The listing builds one solid part. Answer for the finished solid, in the listing's coordinates (mm). Face numbers are marked on the shaded views. A direction names the side the tool comes from. Round coordinates to 2 decimals unless told otherwise and drop trailing zeros.
(1) Find the intervals of material crossed by probe 1 along Y at (x, z) = (5, -12.5); probe 2 along Z at (x, y) = (5, -8.5); probe 3 along Y at (x, z) = (4.5, -1.5), in increasing order.
(2) A cutting plane is placed at A-A, the plane x = 4. Give the number of separate pieces and of enclosed holes in the cut face, and give its area (3 significant figures).
(3) For the marked faces 1 and 2, determine the directions among +Z, -Z, +X, -X, +Y, -Y from which every point of the face is accessible in a straight line to the end or side of a thin tool.
(4) Each of these flat-tipped pins is pushed along its axis until it touches: pin 1 Ø1 at (x, y) = (3, -16.5) entering from -Z; pin 2 Ø1.2 at (x, z) = (4.5, 21) entering from +Y; pin 3 Ø1.2 at (x, z) = (4.5, -16.5) entering from +Y. Where does it stop, or does it pass through?
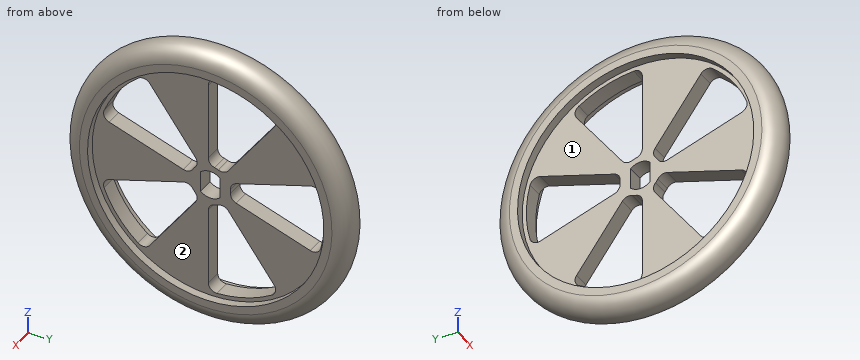
from build123d import *

# Parameters (mm, degrees)
SKETCH1_R                = 31
BOSS_EXTRUDE1_DEPTH      = 8
SKETCH3_R                = 29
CUT_EXTRUDE1_DEPTH       = 2
CUT_EXTRUDE2_DEPTH       = 45.24929378
FILLET2_R                = 2
CIRPATTERN1_COUNT        = 5
FILLET2_OF_CIRPATTERN1_R = 2
CUT_EXTRUDE3_REACH       = 46.249


with BuildPart() as part:
    # Sketch1 → Boss-Extrude1 (new body)
    with BuildSketch(Plane(origin=(0, 0, 0), x_dir=(0, 0, -1), z_dir=(1, 0, 0))):
        Circle(SKETCH1_R)
    extrude(amount=BOSS_EXTRUDE1_DEPTH)

    # Sketch3 → Cut-Extrude1 (cut)
    with BuildSketch(Plane(origin=(8, 0, 0), x_dir=(0, 0, -1), z_dir=(1, 0, 0))):
        Circle(SKETCH3_R)
    cut_extrude1 = extrude(amount=-CUT_EXTRUDE1_DEPTH, mode=Mode.SUBTRACT)

    # Sketch4 → Cut-Extrude2 (cut, through all)
    with BuildSketch(Plane(origin=(6, 0, 0), x_dir=(0, 0, -1), z_dir=(1, 0, 0))):
        with BuildLine():
            Line((-2, 4.582575695), (-9.113404062, 26.475382271))
            ThreePointArc((-9.113404062, 26.475382271), (0, 28), (9.113404062, 26.475382271))
            Line((9.113404062, 26.475382271), (2, 4.582575695))
            ThreePointArc((2, 4.582575695), (0, 5), (-2, 4.582575695))
        make_face()
    cut_extrude2 = extrude(amount=-CUT_EXTRUDE2_DEPTH, mode=Mode.SUBTRACT)

    # Fillet2
    fillet2_edges = [part.edges().sort_by_distance(p)[0] for p in [
        (3, 4.582575695, -2),
        (3, 4.582575695, 2),
        (3, 26.475382271, 9.113404062),
        (3, 26.475382271, -9.113404062),
    ]]
    fillet(fillet2_edges, radius=FILLET2_R)

    # CirPattern1: Cut-Extrude2 ×5 about axis
    cirpattern1_axis = Axis((0, 0, 0), (1, 0, 0))
    for i in range(1, CIRPATTERN1_COUNT):
        add(cut_extrude2.rotate(cirpattern1_axis, i * 360 / CIRPATTERN1_COUNT), mode=Mode.SUBTRACT)

    # Fillet2 of CirPattern1
    fillet2_of_cirpattern1_edges = [part.edges().sort_by_distance(p)[0] for p in [
        (3, 3.3182068, 3.740254487),
        (3, -0.486019265, 4.976322465),
        (3, -0.486019265, 27.995781562),
        (3, 16.848705373, 22.363388098),
        (3, -2.531811111, 4.3116044),
        (3, -4.88295212, 1.075536422),
        (3, -26.775758696, 8.188940485),
        (3, -16.062309684, 22.934738011),
        (3, -4.88295212, -1.075536422),
        (3, -2.531811111, -4.3116044),
        (3, -16.062309684, -22.934738011),
        (3, -26.775758696, -8.188940485),
        (3, -0.486019265, -4.976322465),
        (3, 3.3182068, -3.740254487),
        (3, 16.848705373, -22.363388098),
        (3, -0.486019265, -27.995781562),
    ]]
    fillet(fillet2_of_cirpattern1_edges, radius=FILLET2_OF_CIRPATTERN1_R)

    # Mirror1: Cut-Extrude1 across plane
    add(cut_extrude1.mirror(Plane(origin=(4, 0, 0), x_dir=(0, 0, 1), z_dir=(1, 0, 0))), mode=Mode.SUBTRACT)

    # Sketch5 → Cut-Extrude3 (cut, up to next)
    with BuildSketch(Plane(origin=(6, 0, 0), x_dir=(0, 0, -1), z_dir=(1, 0, 0)), mode=Mode.PRIVATE) as cut_extrude3_sk1:
        with BuildLine():
            Line((-2.547547841, 2.4), (2.547547841, 2.4))
            ThreePointArc((2.547547841, 2.4), (3.5, 0), (2.547547841, -2.4))
            Line((2.547547841, -2.4), (-2.547547841, -2.4))
            ThreePointArc((-2.547547841, -2.4), (-3.5, 0), (-2.547547841, 2.4))
        make_face()
    cut_extrude3_tool1 = extrude(cut_extrude3_sk1.sketch, amount=-CUT_EXTRUDE3_REACH, mode=Mode.PRIVATE) & part.part
    add(cut_extrude3_tool1.solids().sort_by_distance((6, 0, 0))[0], mode=Mode.SUBTRACT)

    # Sketch6 → Revolve1 (revolve)
    with BuildSketch(Plane.XY, mode=Mode.PRIVATE) as revolve1_sk:
        with BuildLine():
            Line((0, 31), (8, 31))
            ThreePointArc((8, 31), (4, 35), (0, 31))
        make_face()
    revolve(revolve1_sk.sketch.rotate(Axis((-0.381, 0, 0), (1, 0, 0)), 90), axis=Axis((-0.381, 0, 0), (1, 0, 0)))


solid = part.part
Solutions:
1. probe 1: y = -32.56 to -25.05, -8.48 to -0.49, 9.68 to 32.56
1. probe 2: z = -33.82 to -12.53, -2.25 to 2.25, 12.53 to 33.82
1. probe 3: y = -34.94 to -2.4, 2.4 to 5.15, 27.96 to 34.94
2. separate pieces: 1
2. enclosed holes: 6
2. area: 2,530 mm2
3. face 1: -X
3. face 2: +X
4. pin 1: stops at z = -31.02
4. pin 2: stops at y = 28.41
4. pin 3: stops at y = 31.15
